Design review of the part built by this model. Coordinates are the model's own, in mm. A direction names the side the tool comes from. Round coordinates to 2 decimals unless told otherwise and drop trailing zeros. Order: outer loops, then holes, each group sorted by start corner. A loop starts at its lowest first (then second) coordinate and runs counter-clockwise, first axis right, second up. Notation, with made-up numbers: (66, 85) - (70, 85) arc R15 cw to (70, 113) - close; hole circle Ø3 at (14, 41). An arc over 180 degrees is marked (long way). Answer as a JSON object with one key per item and string values. Group by question number.
from build123d import *

# Parameters (mm, degrees)
F0_W      = 152.4
F0_H      = 3.175
F1_DEPTH  = 177.8
F2_W      = 152.4
F2_H      = 6.35
F2_H_2    = 6.349996
F3_DEPTH  = 25.4
F4_SIZE   = 12.7
F5_R      = 6.35
F6_DEPTH  = 12.7
F7_R      = 6.35
F8_DEPTH  = 12.7
F9_R      = 50.8
F10_DEPTH = 6.35
F11_R     = 50.8
F12_DEPTH = 6.35


with BuildPart() as f1:
    # F0 (on Front) → F1 (new body, symmetric)
    with BuildSketch(Plane.XZ):
        Rectangle(F0_W, F0_H)
    extrude(amount=F1_DEPTH, both=True)

    # F2 (on Top) → F3 (join, symmetric)
    with BuildSketch(Plane.XY):
        with Locations((0, -174.625)):
            Rectangle(F2_W, F2_H)
        with Locations((0, 174.625002)):
            Rectangle(F2_W, F2_H_2)
    extrude(amount=F3_DEPTH, both=True)

    # F4
    f4_edges = [f1.edges().sort_by_distance(p)[0] for p in [
        (76.2, -174.625, 25.4),
        (-76.2, -174.625, 25.4),
        (-76.2, -174.625, -25.4),
        (76.2, -174.625, -25.4),
        (76.2, 174.625002, 25.4),
        (-76.2, 174.625002, 25.4),
        (76.2, 174.625002, -25.4),
        (-76.2, 174.625002, -25.4),
    ]]
    chamfer(f4_edges, length=F4_SIZE)

    # F5 (on face) → F6 (join)
    with BuildSketch(Plane(origin=(0, 177.8, 0), x_dir=(-1, 0, 0), z_dir=(0, 1, 0))):
        Circle(F5_R)
    extrude(amount=F6_DEPTH)

    # F7 (on face) → F8 (join)
    with BuildSketch(Plane.XZ.offset(177.8)):
        Circle(F7_R)
    extrude(amount=F8_DEPTH)

    # F9 (on face) → F10 (join)
    with BuildSketch(Plane(origin=(0, 177.8, 0), x_dir=(-1, 0, 0), z_dir=(0, 1, 0))):
        Circle(F9_R)
    extrude(amount=-F10_DEPTH)

    # F11 (on face) → F12 (join)
    with BuildSketch(Plane.XZ.offset(177.8)):
        Circle(F11_R)
    extrude(amount=-F12_DEPTH)


solid = f1.part
1. Take a section at C-C, the plane y = 25. Give the boundary of the cut face in (x, z).
2. To check wall thickness, follow line 1 (Y direction, x = -35, z = -3); line 2 (Z direction, x = -6, y = 26). State the ranges of each line that lie inside material, in increasing order. Write a range as from..to.
3. Take a section at D-D, the plane x = 28.5. Give the boundary of the cut face in (y, z), then the cut area to 3 significant figures.
4. Clearance check with flat-ended pins moving along their axes: P1, Ø5, axis at x = -57, z = -16.5, coming from the -Y side; P2, Ø8, axis at x = -17.5, y = 91.5, coming from the -Z side; P3, Ø1.9, axis at x = -53, y = 173, coming from the -Z side; P4, Ø8, axis at y = 75, z = -6, coming from the -X side. State where each tip first meets the part, or that it passes through.
5. Take a section at B-B, the plane x = 0. Give the boundary of the cut face in (y, z), then the cut area to 3 significant figures.
6. Take a section at A-A, the plane z = -31.5. Give the boundary of the cut face in (x, y).
7. Tool access review of faces 1 (the flat face through (-54, -175, 25.4)), 2 (the flat face through (-60, 171.45, -13)), 3 (the flat face through (-54, -175, -25.4)): name each direction out of +Z, -Z, +X, -X, +Y, -Y from which nothing blocks a thin tool from reaching the whole face with its end or side.
8. Mouldability with a two-part tool opening along Y and no side actions: class faces 4 (the flat face through (-54, 175, -25.4)), 5 (the flat face through (1, 171.45, -20)) as pulls with the +Y half, pulls with the -Y half, needs draft (parallel to the pull), parting line crosses it, or undercut.
Response values:
{
 "1": {"outline": "(-76.2, -1.59) - (76.2, -1.59) - (76.2, 1.59) - (-76.2, 1.59) - close"},
 "2": {"line 1": "-177.8..-171.45, 171.45..177.8", "line 2": "-1.59..1.59"},
 "3": {"outline": "(-177.8, -42.05) - (-171.45, -42.05) - (-171.45, -1.59) - (171.45, -1.59) - (171.45, -42.05) - (177.8, -42.05) - (177.8, 42.05) - (171.45, 42.05) - (171.45, 1.59) - (-171.45, 1.59) - (-171.45, 42.05) - (-177.8, 42.05) - close", "area": "2,160 mm2"},
 "4": {"P1": "y = -177.8", "P2": "z = -1.59", "P3": "z = -25.4", "P4": "through"},
 "5": {"outline": "(-190.5, -6.35) - (-177.8, -6.35) - (-177.8, -50.8) - (-171.45, -50.8) - (-171.45, -1.59) - (171.45, -1.59) - (171.45, -50.8) - (177.8, -50.8) - (177.8, -6.35) - (190.5, -6.35) - (190.5, 6.35) - (177.8, 6.35) - (177.8, 50.8) - (171.45, 50.8) - (171.45, 1.59) - (-171.45, 1.59) - (-171.45, 50.8) - (-177.8, 50.8) - (-177.8, 6.35) - (-190.5, 6.35) - close", "area": "2,700 mm2"},
 "6": {"outline": "(-39.85, -177.8) - (39.85, -177.8) - (39.85, -171.45) - (-39.85, -171.45) - close; (-39.85, 171.45) - (39.85, 171.45) - (39.85, 177.8) - (-39.85, 177.8) - close"},
 "7": {"face 1": "+Z, -X, +Y, -Y", "face 2": "-Z, +X, -X", "face 3": "-Z, -X, +Y, -Y"},
 "8": {"face 4": "needs draft", "face 5": "undercut"}
}
